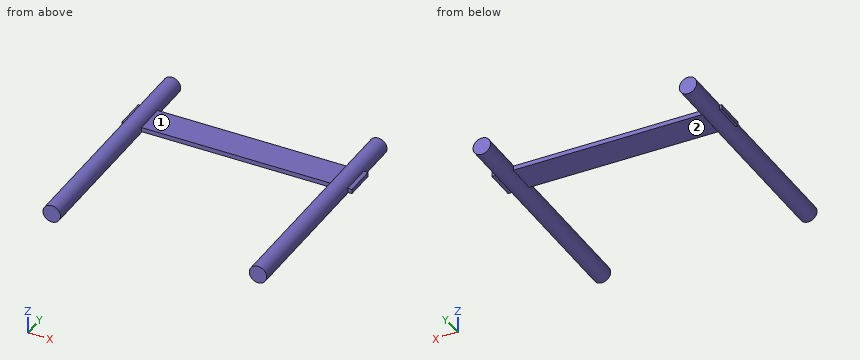
```python
from build123d import *

# Parameters (mm, degrees)
F0_R     = 50
F1_DEPTH = 655
F2_W     = 1314.7466778755
F2_H     = 174.9388724566
F3_DEPTH = 12.5


with BuildPart() as f1:
    # F0 (on Front) → F1 (new body, symmetric)
    with BuildSketch(Plane.XZ):
        with Locations((590, 0)):
            Circle(F0_R)
    extrude(amount=F1_DEPTH, both=True)



with BuildPart() as f1b:
    # F0 (on Front) → F1, piece 2 (new body, symmetric)
    with BuildSketch(Plane.XZ):
        with Locations((-590, 0)):
            Circle(F0_R)
    extrude(amount=F1_DEPTH, both=True)


with BuildPart() as f1_1:
    add(f1.part)

    add(f1b.part)  # F3 merges F1b
    # F2 (on Top) → F3 (join, symmetric)
    with BuildSketch(Plane.XY):
        with Locations((5.4104626179, 317.414842546)):
            Rectangle(F2_W, F2_H)
    extrude(amount=F3_DEPTH, both=True)


solid = f1_1.part
```
Check sheet for the modelled part. Datum: model origin and axes. Units: mm. Face numbers are marked on the shaded views. A direction names the side the tool comes from. Give positions to 0.01 mm unless a question says otherwise; leave off trailing zeros. Loops run counter-clockwise (first coordinate to the right, second up) from the corner with the lowest first, then second, coordinate; pieces in that order, holes last. Notation, with made-up numbers: M 36.5,-32 L 55.5,-32 A8 cw 55.5,-22 Z; hole C 51.5,35 d4. An arc over 180 degrees is marked long. Answer as CSV lines item,"result".
Item 1: Scan lines: L1, parallel to X at y = 585, z = -5.5; L2, parallel to X at y = 138, z = -13.5; L3, parallel to Z at x = 594, y = -51.5. Record each from-to range of solid material in increasing order.
Reply:
L1,"-639.7 to -540.3, 540.3 to 639.7"
L2,"-638.14 to -541.86, 541.86 to 638.14"
L3,"-49.84 to 49.84"
Item 2: Sectioned sample at B-B, the plane y = -128. Enter the section's corners in (x, z), then the cut area to 3 significant figures.
Reply:
outline,"C -590,0 d100; C 590,0 d100"
area,"15,700 mm^2"
Item 3: Set-up check for the marked faces 1 and 2: record each of +Z, -Z, +X, -X, +Y, -Y from which the full face is reachable in a straight line by a thin tool's end or side.
Reply:
face 1,"+Z, +Y, -Y"
face 2,"-Z, +Y, -Y"
Item 4: Sectioned sample at C-C, the plane x = -167.5. Enter the section's corners in (y, z).
Reply:
outline,"M 229.95,-12.5 L 404.88,-12.5 L 404.88,12.5 L 229.95,12.5 Z"
Item 5: Sectioned sample at D-D, the plane x = 564. Enter the section's corners in (y, z), then the cut area to 3 significant figures.
Reply:
outline,"M -655,-42.71 L 655,-42.71 L 655,42.71 L -655,42.71 Z"
area,"112,000 mm^2"
Item 6: Sectioned sample at A-A, the plane y = 285.5. Enter the section's corners in (x, z).
Reply:
outline,"M -651.96,-12.5 L -638.41,-12.5 A50 ccw -541.59,-12.5 L 541.59,-12.5 A50 ccw 638.41,-12.5 L 662.78,-12.5 L 662.78,12.5 L 638.41,12.5 A50 ccw 541.59,12.5 L -541.59,12.5 A50 ccw -638.41,12.5 L -651.96,12.5 Z"
Item 7: Depth check by flat-ended pin: pin 1 Ø8 at (y, z) = (-336, 23) entering from -X; pin 2 Ø20 at (x, z) = (-116, 2.5) entering from -Y; pin 3 Ø3 at (x, z) = (-301, 9) entering from +Y. Enter the tip coordinate at first touch or a pass-through.
Reply:
pin 1,"x = -636.25"
pin 2,"y = 229.95"
pin 3,"y = 404.88"
